Model file for the job. Use its own axes, mm. A direction names the side the tool comes from. Round coordinates to 2 decimals unless told otherwise and drop trailing zeros. Order: outer loops, then holes, each group sorted by start corner. A loop starts at its lowest first (then second) coordinate and runs counter-clockwise, first axis right, second up. Notation, with made-up numbers: (18, 17) -> (52, 17) arc R20 cw to (52, 50) -> close; hole circle Ø3 at (61.25, -30). An arc over 180 degrees is marked (long way). Answer as CSV lines item,"result".
```python
from build123d import *

# Parameters (mm, degrees)
ESQUISSE1_R             = 16
BOSS_EXTRU_1_DEPTH      = 22
ESQUISSE2_W             = 2.8
ESQUISSE2_H             = 31
ENL_V_MAT_EXTRU_1_DEPTH = 11.41
ESQUISSE3_W             = 2.8
ESQUISSE3_H             = 1.9
BOSS_EXTRU_2_DEPTH      = 5
ESQUISSE4_R             = 14
ENL_V_MAT_EXTRU_2_DEPTH = 18


with BuildPart() as part:
    # Esquisse1 → Boss.-Extru.1 (new body)
    with BuildSketch(Plane.XY):
        Circle(ESQUISSE1_R)
    extrude(amount=BOSS_EXTRU_1_DEPTH)

    # Esquisse2 → Enlèv. mat.-Extru.1 (cut)
    with BuildSketch(Plane.XY):
        Rectangle(ESQUISSE2_W, ESQUISSE2_H)
    extrude(amount=ENL_V_MAT_EXTRU_1_DEPTH, mode=Mode.SUBTRACT)

    # Esquisse3 → Boss.-Extru.2 (add)
    with BuildSketch(Plane(origin=(0, 0, 0), x_dir=(-1, 0, 0), z_dir=(0, 0, -1))):
        with Locations((0, -6.25)):
            Rectangle(ESQUISSE3_W, ESQUISSE3_H)
        with Locations((0, 3.95)):
            Rectangle(ESQUISSE3_W, ESQUISSE3_H)
    extrude(amount=-BOSS_EXTRU_2_DEPTH)

    # Esquisse4 → Enlèv. mat.-Extru.2 (cut)
    with BuildSketch(Plane.XY.offset(22)):
        Circle(ESQUISSE4_R)
    extrude(amount=-ENL_V_MAT_EXTRU_2_DEPTH, mode=Mode.SUBTRACT)


solid = part.part
```
Q1. Saw through at B-B (x = 0). Write the cut outline in (y, z), plus the area to 3 significant figures.
Checks:
outline,"(-16, 0) -> (-15.5, 0) -> (-15.5, 11.41) -> (-14, 11.41) -> (-14, 22) -> (-16, 22) -> close; (-7.2, 0) -> (-5.3, 0) -> (-5.3, 4) -> (-7.2, 4) -> close; (3, 0) -> (4.9, 0) -> (4.9, 4) -> (3, 4) -> close; (14, 11.41) -> (15.5, 11.41) -> (15.5, 0) -> (16, 0) -> (16, 22) -> (14, 22) -> close"
area,"69.0 mm²"
Q2. Saw through at C-C (z = 11). Write the cut outline in (x, y).
Checks:
outline,"circle Ø32 at (0, 0); hole (-1.4, -15.5) -> (1.4, -15.5) -> (1.4, -13.93) arc R14 ccw to (1.4, 13.93) -> (1.4, 15.5) -> (-1.4, 15.5) -> (-1.4, 13.93) arc R14 ccw to (-1.4, -13.93) -> close"
Q3. Mould opens along Y. For faces 1 (the cylindrical face through (-3.47, -15.62, 10.85)), 2 (the flat face through (0, -15, 11.41)), 3 (the flat face through (3, 0, 0)) say: +Y half, -Y half, draft (parallel to the pull), parting line (faces both ways), or undercut.
Checks:
face 1,"parting line"
face 2,"undercut"
face 3,"draft"
Q4. Wall check: L1, parallel to Y at x = -0.5, z = 10; L2, parallel to Y at x = 0, z = 12.25; L3, parallel to Z at x = -12, y = 0.5. Give the ranges that are in metal, low to high. Write a range as [from, to].
Checks:
L1,"[-15.99, -15.5], [15.5, 15.99]"
L2,"[-16, -14], [14, 16]"
L3,"[0, 4]"
Q5. Saw through at D-D (x = 4). Write the cut outline in (y, z), plus the area to 3 significant figures.
Checks:
outline,"(-15.49, 0) -> (15.49, 0) -> (15.49, 22) -> (13.42, 22) -> (13.42, 4) -> (-13.42, 4) -> (-13.42, 22) -> (-15.49, 22) -> close"
area,"199 mm²"
Q6. Tool access for faces 4 (the flat face through (-0.07, -14.15, 22)), 5 (the cylindrical face through (12.932, -5.362, 13.126)), 6 (the flat face through (1.4, 11, 3)), 7 (the flat face through (0, -5.3, 2)): list every direction of +Z, -Z, +X, -X, +Y, -Y with a clear straight run to the whole face (end or side of a thin tool).
Checks:
face 4,"+Z, +X, -X, +Y, -Y"
face 5,"+Z"
face 6,"-Z"
face 7,"+Z, -Z"
Q7. Flat gauge pins, fed straight in: pin 1 (5 mm diameter, centred on y = 10, z = 14.5, fed in from -X); pin 2 (5.5 mm diameter, centred on y = 7.5, z = 7.5, fed in from +X); pin 3 (3 mm diameter, centred on y = 10.5, z = 2.5, fed in from -X). Where does each tip first touch, or does it go through?
Checks:
pin 1,"x = -14.13"
pin 2,"x = 15.28"
pin 3,"x = -13.23"
Q8. Saw through at A-A (y = 0). Write the cut outline in (x, z), plus the area to 3 significant figures.
Checks:
outline,"(-16, 0) -> (-1.4, 0) -> (-1.4, 4) -> (-14, 4) -> (-14, 22) -> (-16, 22) -> close; (1.4, 0) -> (16, 0) -> (16, 22) -> (14, 22) -> (14, 4) -> (1.4, 4) -> close"
area,"189 mm²"
